Design review of the part built by this model. Coordinates are the model's own, in mm. A direction names the side the tool comes from. Coordinates: 2 decimals unless noted, no trailing zeros. Write each loop counter-clockwise with the first axis right and the second up, starting at its lowest first coordinate (ties: lowest second). Pieces come first, ordered by that corner, then holes. Notation, with made-up numbers: (-18, -33.5) -> (32, -33.5) arc R31 cw to (32, 1.5) -> close; hole circle Ø5 at (21, 54). An arc over 180 degrees is marked (long way). Write item = value, one per line. Start each with the question number.
```python
from build123d import *

# Parameters (mm, degrees)
SKETCH_1_W           = 50
SKETCH_1_H           = 28
EXTRUDE_1_DEPTH      = 6
CUT_EXTRUDE_1_DEPTH  = 1
FILLET_3_R           = 0.5
SKETCH_5_OUTSIDE_W   = 63.524
SKETCH_5_OUTSIDE_H   = 41.524
SKETCH_5_OUTSIDE_W_2 = 40
SKETCH_5_OUTSIDE_H_2 = 13
CUT_EXTRUDE_2_DEPTH  = 4
FILLET_1_R           = 0.5
SKETCH_6_W           = 39
SKETCH_6_H           = 12
EXTRUDE_2_DEPTH      = 0.3


with BuildPart() as part:
    # 草图1 → 凸台-拉伸1 (new body)
    with BuildSketch(Plane(origin=(0, 0, 0), x_dir=(1, 0, 0), z_dir=(0, 1, 0))):
        with Locations((23, -12)):
            Rectangle(SKETCH_1_W, SKETCH_1_H)
    extrude(amount=EXTRUDE_1_DEPTH)

    # 草图3 → 切除-拉伸1 (cut)
    with BuildSketch(Plane(origin=(0, 6, 0), x_dir=(1, 0, 0), z_dir=(0, 1, 0))):
        Polygon((-0.5, 0.5), (8, 0.5), (8, 0.1), (38, 0.1), (38, 0.5), (46.5, 0.5), (46.5, -8), (46.1, -8), (46.1, -16), (46.5, -16), (46.5, -24.5), (38, -24.5), (38, -24.1), (8, -24.1), (8, -24.5), (-0.5, -24.5), (-0.5, -16), (-0.1, -16), (-0.1, -8), (-0.5, -8), align=None)
    extrude(amount=-CUT_EXTRUDE_1_DEPTH, mode=Mode.SUBTRACT)

    # 圆角3
    # the kernel refuses this fillet: 0.5 mm, written as the material it adds along each edge
    with BuildSketch(Plane(origin=(38, 6, -0.5), x_dir=(1.6520118606416786e-12, 0, 1.0), z_dir=(0, -1, 0)), Plane(origin=(46.5, 6, 16), x_dir=(-1.0, 0, 1.5276668818837323e-12), z_dir=(0, -1, 0)), Plane(origin=(8, 6, 24.5), x_dir=(-1.5765166949672239e-12, 0, -1.0), z_dir=(0, -1, 0)), Plane(origin=(-0.5, 6, 8), x_dir=(1.0, 0, -1.5831780331149617e-12), z_dir=(0, -1, 0))) as fillet_3_piece_1:
        with BuildLine():
            CenterArc((0.5, -0.489897949), FILLET_3_R, 101.536959033, 78.463040967)
            Line((0, -0.489897949), (-0.01, -0.489897949))
            Line((-0.01, -0.489897949), (-0.01, 0))
            Line((-0.01, 0), (0, 0.01))
            ThreePointArc((0, 0.01), (0.2, 0.01), (0.398, 0.009797959))
            Line((0.398, 0.009797959), (0.4, 0))
        make_face()
    extrude(amount=2.224744871)
    with BuildSketch(Plane(origin=(46.5, 6, 8), x_dir=(0, 0, -1), z_dir=(0, -1, 0)), Plane(origin=(38, 6, 24.5), x_dir=(1, 0, 0), z_dir=(0, -1, 0)), Plane(origin=(-0.5, 6, 16), x_dir=(0, 0, 1), z_dir=(0, -1, 0)), Plane(origin=(8, 6, -0.5), x_dir=(-1, 0, 0), z_dir=(0, -1, 0))) as fillet_3_piece_2:
        with BuildLine():
            CenterArc((0.489897949, -0.5), FILLET_3_R, 90, 78.463040967)
            Line((0, -0.4), (-0.009797959, -0.398))
            ThreePointArc((-0.009797959, -0.398), (-0.01, -0.2), (-0.01, 0))
            Line((-0.01, 0), (0, 0.01))
            Line((0, 0.01), (0.489897949, 0.01))
            Line((0.489897949, 0.01), (0.489897949, 0))
        make_face()
    extrude(amount=2.224744871)
    with BuildSketch(Plane(origin=(46.5, 6, -0.5), x_dir=(-1, 0, 0), z_dir=(0, -1, 0)), Plane(origin=(46.5, 6, 24.5), x_dir=(0, 0, -1), z_dir=(0, -1, 0)), Plane(origin=(-0.5, 6, 24.5), x_dir=(1, 0, 0), z_dir=(0, -1, 0))) as fillet_3_piece_3:
        with BuildLine():
            CenterArc((FILLET_3_R, -FILLET_3_R), FILLET_3_R, 90, 90)
            Line((0, -FILLET_3_R), (-FILLET_3_R * 0.02, -FILLET_3_R))
            Line((-FILLET_3_R * 0.02, -FILLET_3_R), (-FILLET_3_R * 0.02, FILLET_3_R * 0.02))
            Line((-FILLET_3_R * 0.02, FILLET_3_R * 0.02), (FILLET_3_R, FILLET_3_R * 0.02))
            Line((FILLET_3_R, FILLET_3_R * 0.02), (FILLET_3_R, 0))
        make_face()
    extrude(amount=2.25)
    with BuildSketch(Plane(origin=(-0.5, 6, -0.5), x_dir=(1, 0, 0), z_dir=(0, -1, 0))) as fillet_3_piece_4:
        with BuildLine():
            CenterArc((FILLET_3_R, FILLET_3_R), FILLET_3_R, 180, 90)
            Line((0, FILLET_3_R), (-FILLET_3_R * 0.02, FILLET_3_R))
            Line((-FILLET_3_R * 0.02, FILLET_3_R), (-FILLET_3_R * 0.02, -FILLET_3_R * 0.02))
            Line((-FILLET_3_R * 0.02, -FILLET_3_R * 0.02), (FILLET_3_R, -FILLET_3_R * 0.02))
            Line((FILLET_3_R, -FILLET_3_R * 0.02), (FILLET_3_R, 0))
        make_face()
    extrude(amount=2.25)

    # 草图5 outside → 切除-拉伸2 (cut)
    with BuildSketch(Plane(origin=(0, 0, 0), x_dir=(-1, 0, 0), z_dir=(0, -1, 0))):
        with Locations((-23, -12)):
            Rectangle(SKETCH_5_OUTSIDE_W, SKETCH_5_OUTSIDE_H)
        with Locations((-23, -12)):
            Rectangle(SKETCH_5_OUTSIDE_W_2, SKETCH_5_OUTSIDE_H_2, mode=Mode.SUBTRACT)
    extrude(amount=-CUT_EXTRUDE_2_DEPTH, mode=Mode.SUBTRACT)

    # 圆角1
    fillet_1_edges = [part.edges().sort_by_distance(p)[0] for p in [
        (43, 2, 5.5),
        (3, 2, 5.5),
        (3, 2, 18.5),
        (43, 2, 18.5),
        (-2, 5, -2),
        (48, 5, -2),
        (48, 5, 26),
        (-2, 5, 26),
    ]]
    fillet(fillet_1_edges, radius=FILLET_1_R)

    # 草图6 → 凸台-拉伸2 (add)
    with BuildSketch(Plane(origin=(0, 5, 0), x_dir=(1, 0, 0), z_dir=(0, 1, 0))):
        with Locations((23, -12)):
            Rectangle(SKETCH_6_W, SKETCH_6_H)
    extrude(amount=EXTRUDE_2_DEPTH)


solid = part.part
```
(1) For line 1 (Z direction, x = 25, y = 5.1); line 2 (X direction, y = 5.05, z = 5.25); line 3 (Y direction, x = 32.5, z = 13.25), list the stretches that pass through material, from the lowest coordinate up.
(2) Take a section at C-C, the plane x = 23.5. State the section outline as (y, z) points.
(3) For faces 4 (the face through (-0.1, 5.5, 12.1)), 5 (the face through (23, 0, 12)), 6 (the face through (48, 5, 12)), 7 (the face through (3, 2, 12)), 8 (the face through (23, 2, 5.5)), list the 3-axis set-ups (+Z, -Z, +X, -X, +Y, -Y) from which the entire face can be reached by the end or side of a thin tool; tool diameter is ignored.
(4) Take a section at B-B, the plane y = 2.5. State the section outline as (x, z) points, then the cut area to 3 significant figures.
(5) For pin 1 Ø6 at (x, z) = (28.5, 13.5) entering from +Y; pin 2 Ø1.5 at (x, y) = (19, 0.5) entering from -Z; pin 3 Ø1.5 at (y, z) = (2.5, 5.5) entering from -X, all flat-tipped, find the tip position at first contact; note any pin that passes through.
(6) Mouldability with a two-part tool opening along X and no side actions: class faces 1 (the face through (43, 2, 12)), 2 (the face through (23, 5, 26)), 3 (the face through (23, 5, 3)) as pulls with the +X half, pulls with the -X half, needs draft (parallel to the pull), parting line crosses it, or undercut.
(7) Take a section at D-D, the plane z = 1.75. State the section outline as (x, y) points.
(8) Take a section at A-A, the plane z = 10.5. State the section outline as (x, y) points, then the cut area to 4 significant figures.
Report:
q1.line_1 = -2 to -0.1, 6 to 18, 24.1 to 26
q1.line_2 = -2 to -0.5, 46.5 to 48
q1.line_3 = 0 to 5.3
q2.outline = (0, 5.5) -> (4, 5.5) -> (4, -2) -> (6, -2) -> (6, -0.1) -> (5, -0.1) -> (5, 6) -> (5.3, 6) -> (5.3, 18) -> (5, 18) -> (5, 24.1) -> (6, 24.1) -> (6, 26) -> (4, 26) -> (4, 18.5) -> (0, 18.5) -> close
q3.face_4 = +Y
q3.face_5 = +Z, -Z, +X, -X, -Y
q3.face_6 = +Z, -Z, +X, +Y, -Y
q3.face_7 = +Z, -Z, -X, -Y
q3.face_8 = -Z, +X, -X, -Y
q4.outline = (3, 6) arc R0.5 ccw to (3.5, 5.5) -> (42.5, 5.5) arc R0.5 ccw to (43, 6) -> (43, 18) arc R0.5 ccw to (42.5, 18.5) -> (3.5, 18.5) arc R0.5 ccw to (3, 18) -> close
q4.area = 520 mm2
q5.pin_1 = 5.3
q5.pin_2 = 5.5
q5.pin_3 = 3
q6.face_1 = pulls with the +X half
q6.face_2 = needs draft
q6.face_3 = undercut
q7.outline = (-2, 4) -> (48, 4) -> (48, 6) -> (46.5, 6) -> (46.5, 5) -> (-0.5, 5) -> (-0.5, 6) -> (-2, 6) -> close
q8.outline = (-2, 4) -> (3, 4) -> (3, 0) -> (43, 0) -> (43, 4) -> (48, 4) -> (48, 6) -> (46.1, 6) -> (46.1, 5) -> (42.5, 5) -> (42.5, 5.3) -> (3.5, 5.3) -> (3.5, 5) -> (-0.1, 5) -> (-0.1, 6) -> (-2, 6) -> close
q8.area = 225.5 mm2
